Geometry check sheet. Reference: the model listing, model coordinates, mm. A direction names the side the tool comes from. Round coordinates to 2 decimals unless told otherwise and drop trailing zeros. Loops run counter-clockwise (first coordinate to the right, second up) from the corner with the lowest first, then second, coordinate; pieces in that order, holes last. Notation, with made-up numbers: (-21.75, 40.25) -> (-4.75, 40.25) arc R13 cw to (-4.75, 59.25) -> close; hole circle Ø4 at (53, 89.25). An arc over 180 degrees is marked (long way). Use one line per item in the form item = value.
from build123d import *

# Parameters (mm, degrees)
SKETCH_1_R          = 2.5
SKETCH_1_R_2        = 2.05
EXTRUDE_1_DEPTH     = 5
SKETCH_2_R          = 2.5
EXTRUDE_2_DEPTH     = 5
FILLET_1_R          = 6
FILLET_2_R          = 10
SKETCH_3_R          = 1.6
EXTRUDE_3_DEPTH     = 5
FILLET_3_R          = 10
SKETCH_4_W          = 47.859617289
SKETCH_4_H          = 15
CUT_EXTRUDE_1_DEPTH = 6.0000001
SKETCH_6_R          = 2.65
CUT_EXTRUDE_2_DEPTH = 1.4
EXTRUDE_5_DEPTH     = 5
SKETCH_11_R         = 4.525
CUT_EXTRUDE_4_DEPTH = 6.0000001
SKETCH_13_R         = 5.06
CUT_EXTRUDE_5_DEPTH = 5


with BuildPart() as part:
    # 草图1 → 凸台-拉伸1 (new body)
    with BuildSketch(Plane(origin=(0, 0, 0), x_dir=(0, 0, -1), z_dir=(1, 0, 0))):
        with BuildLine():
            Line((0, 5), (90, 5))
            ThreePointArc((90, 5), (95, 0), (90, -5))
            Line((90, -5), (0, -5))
            ThreePointArc((0, -5), (-5, 0), (0, 5))
        make_face()
        Circle(SKETCH_1_R, mode=Mode.SUBTRACT)
        with Locations((90, 0)):
            Circle(SKETCH_1_R_2, mode=Mode.SUBTRACT)
    extrude(amount=EXTRUDE_1_DEPTH)

    # 草图2 → 凸台-拉伸2 (add)
    with BuildSketch(Plane(origin=(5, 0, 0), x_dir=(0, 0, -1), z_dir=(1, 0, 0))):
        with BuildLine():
            Line((49.91480075, 7.043176995), (48.200371687, 5))
            Line((48.200371687, 5), (36.190624625, 5))
            Line((36.190624625, 5), (42.867191873, 12.956823005))
            ThreePointArc((42.867191873, 12.956823005), (49.347819316, 13.523804438), (49.91480075, 7.043176995))
        make_face()
        with Locations((46.390996312, 10)):
            Circle(SKETCH_2_R, mode=Mode.SUBTRACT)
    extrude(amount=-EXTRUDE_2_DEPTH)

    # 圆角1
    fillet_1_edges = [part.edges().sort_by_distance(p)[0] for p in [
        (2.5, 5, -48.200371687),
    ]]
    fillet(fillet_1_edges, radius=FILLET_1_R)

    # 圆角2
    fillet_2_edges = [part.edges().sort_by_distance(p)[0] for p in [
        (2.5, 5, -36.190624625),
    ]]
    fillet(fillet_2_edges, radius=FILLET_2_R)

    # 草图3 → 凸台-拉伸3 (add)
    with BuildSketch(Plane(origin=(5, 0, 0), x_dir=(0, 0, -1), z_dir=(1, 0, 0))):
        with BuildLine():
            Line((-4.615384615, 1.923076923), (0.384615385, 13.923076923))
            ThreePointArc((0.384615385, 13.923076923), (6.923076923, 16.615384615), (9.615384615, 10.076923077))
            Line((9.615384615, 10.076923077), (7.5, 5))
            Line((7.5, 5), (0, 5))
            ThreePointArc((0, 5), (-2.773500981, 4.160251472), (-4.615384615, 1.923076923))
        make_face()
        with Locations((5, 12)):
            Circle(SKETCH_3_R, mode=Mode.SUBTRACT)
    extrude(amount=-EXTRUDE_3_DEPTH)

    # 圆角3
    fillet_3_edges = [part.edges().sort_by_distance(p)[0] for p in [
        (2.5, 5, -7.5),
    ]]
    fillet(fillet_3_edges, radius=FILLET_3_R)

    # 草图4 → 切除-拉伸1 (cut, through all)
    with BuildSketch(Plane(origin=(5, 0, 0), x_dir=(0, 0, -1), z_dir=(1, 0, 0))):
        with Locations((49.542051895, 12.5)):
            Rectangle(SKETCH_4_W, SKETCH_4_H)
    extrude(amount=-CUT_EXTRUDE_1_DEPTH, mode=Mode.SUBTRACT)

    # 草图6 → 切除-拉伸2 (cut)
    with BuildSketch(Plane(origin=(5, 0, 0), x_dir=(0, 0, -1), z_dir=(1, 0, 0))):
        with Locations((5, 12)):
            Circle(SKETCH_6_R)
    extrude(amount=-CUT_EXTRUDE_2_DEPTH, mode=Mode.SUBTRACT)

    # 草图10 → 凸台-拉伸5 (add)
    with BuildSketch(Plane(origin=(5, 0, 0), x_dir=(0, 0, -1), z_dir=(1, 0, 0))):
        with BuildLine():
            Line((89.732959314, 7.495244444), (19.696938457, 5))
            Line((19.696938457, 5), (90, 5))
            ThreePointArc((90, 5), (95, 0), (90, -5))
            Line((90, -5), (0, -5))
            ThreePointArc((0, -5), (-4.160251472, -2.773500981), (-4.615384615, 1.923076923))
            Line((-4.615384615, 1.923076923), (0.384615385, 13.923076923))
            ThreePointArc((0.384615385, 13.923076923), (0.591982965, 14.359954623), (0.840585507, 14.774756039))
            Line((0.840585507, 14.774756039), (-6.23912174, 4.162134058))
            ThreePointArc((-6.23912174, 4.162134058), (-6.613093279, -3.537936868), (0, -7.5))
            Line((0, -7.5), (90, -7.5))
            ThreePointArc((90, -7.5), (97.498811017, 0.133541513), (89.732959314, 7.495244444))
        make_face()
    extrude(amount=-EXTRUDE_5_DEPTH)

    # 草图11 → 切除-拉伸4 (cut, through all)
    with BuildSketch(Plane(origin=(5, 0, 0), x_dir=(0, 0, -1), z_dir=(1, 0, 0))):
        with Locations((90, 0)):
            Circle(SKETCH_11_R)
    extrude(amount=-CUT_EXTRUDE_4_DEPTH, mode=Mode.SUBTRACT)

    # 草图13 → 切除-拉伸5 (cut)
    with BuildSketch(Plane(origin=(5, 0, 0), x_dir=(0, 0, -1), z_dir=(1, 0, 0))):
        Circle(SKETCH_13_R)
    extrude(amount=-CUT_EXTRUDE_5_DEPTH, mode=Mode.SUBTRACT)


solid = part.part
1. Tool access check on faces 5 (the flat face through (3.6, 12, -7)), 6 (the cylindrical face through (2.535, -3.438, 6.666)). Record the directions out of +Z, -Z, +X, -X, +Y, -Y that give a thin tool (end or side, any length) a straight path to the whole face; none if there is none.
Return value:
face_5 = +X
face_6 = +Z, +X, -X
2. Section check B-B (x = 2.5). Count the separate pieces of the cut face and the enclosed holes in it, then the cut area to 3 significant figures.
Return value:
separate_pieces = 1
enclosed_holes = 3
area = 1,380 mm2
3. Section check C-C (z = -88.5). Record the boundary of the cut face in (x, y), then the cut area to 3 significant figures.
Return value:
outline = (0, -7.5) -> (5, -7.5) -> (5, -4.27) -> (0, -4.27) -> close; (0, 4.27) -> (5, 4.27) -> (5, 7.45) -> (0, 7.45) -> close
area = 32.1 mm2
4. Section check D-D (z = -29). Record the boundary of the cut face in (x, y), then the cut area to 3 significant figures.
Return value:
outline = (0, -7.5) -> (5, -7.5) -> (5, 5.33) -> (0, 5.33) -> close
area = 64.2 mm2
5. Section check A-A (y = 0). Record the boundary of the cut face in (x, z) (3 decimals).
Return value:
outline = (0, -97.5) -> (5, -97.5) -> (5, -94.525) -> (0, -94.525) -> close; (0, -85.475) -> (5, -85.475) -> (5, -5.06) -> (0, -5.06) -> close; (0, 5.06) -> (5, 5.06) -> (5, 7.5) -> (0, 7.5) -> close
6. Material ranges on line 1 along Z through (x, y) = (2.4, -0.25); line 2 along Z through (x, y) = (4.2, -2.5); line 3 along Y through (x, z) = (1.1, 0), recorded low to high.
Return value:
line_1 = -97.5 to -94.52, -85.48 to -5.05, 5.05 to 7.5
line_2 = -97.07 to -93.77, -86.23 to -4.4, 4.4 to 7.07
line_3 = -7.5 to -5.06, 5.06 to 13.51
7. Mould release check, pull along Y, two halves, no side actions. Record for faces 1 (the flat face through (2.54, 9.54, 2.65)), 2 (the flat face through (5, -1, -44)), 3 (the cylindrical face through (2.535, 1.359, -94.316)), 4 (the cylindrical face through (4.31, 9.649, -6.223)): released by +Y, released by -Y, zero draft, split by the parting line, or undercut.
Return value:
face_1 = released by +Y
face_2 = zero draft
face_3 = undercut
face_4 = undercut
8. Gauge pin test, flat ends, axial feed: pin 1 (1 mm diameter, centred on x = 4, z = -38.5, fed in from +Y); pin 2 (2.5 mm diameter, centred on y = 12, z = -5, fed in from -X); pin 3 (8 mm diameter, centred on y = -2.5, z = -68.5, fed in from -X); pin 4 (2 mm diameter, centred on x = 1, y = 3, fed in from +Z). Record the tip position at first contact, or that the pin passes through.
Return value:
pin_1 = 5.69
pin_2 = through
pin_3 = 0
pin_4 = 7.23
